The model under review builds one solid part; all positions refer to its coordinate system, in mm. Face numbers are marked on the shaded views. A direction names the side the tool comes from. Round coordinates to 2 decimals unless told otherwise and drop trailing zeros. Write each loop counter-clockwise with the first axis right and the second up, starting at its lowest first coordinate (ties: lowest second). Pieces come first, ordered by that corner, then holes. Notation, with made-up numbers: (46.25, 67) -> (80.25, 67) arc R23 ccw to (80.25, 81) -> close; hole circle Ø2 at (-21.75, 5). An arc over 180 degrees is marked (long way). Return JSON: item names as keys, results as strings. Group by question number.
1. Tool access review of the marked faces 1 and 2: name each direction out of +Z, -Z, +X, -X, +Y, -Y from which nothing blocks a thin tool from reaching the whole face with its end or side.
2. Take a section at A-A, the plane x = -16. Write out the cut boundary in (y, z).
3. Take a section at C-C, the plane x = -9. Write out the cut boundary in (y, z).
4. Take a section at B-B, the plane y = 15.5. Write out the cut boundary in (x, z).
5. Take a section at D-D, the plane z = 55.5. Write out the cut boundary in (x, y).
6. Clearance check with flat-ended pins moving along their axes: P1, Ø1.5, axis at y = 2, z = 15.5, coming from the +X side; P2, Ø10, axis at x = 13.5, z = 36.5, coming from the -Y side; P3, Ø5, axis at y = 10, z = 28.5, coming from the -X side. State where each tip first meets the part, or that it passes through.
7. For line 1 along Y through (x, z) = (-18.5, 3); line 2 along Z through (x, y) = (-18, -6.5); line 3 along X through (y, z) = (12.5, 23.5), list the stretches that pass through material, from the lowest coordinate up. Write a range as from..to.
8. Mouldability with a two-part tool opening along X and no side actions: class the marked faces 3, 4, 5 and 6 as pulls with the +X half, pulls with the -X half, needs draft (parallel to the pull), parting line crosses it, or undercut.
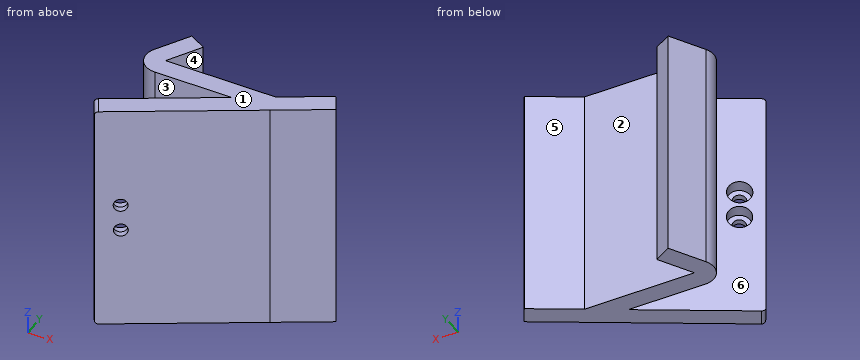
from build123d import *

# Parameters (mm, degrees)
SKETCH_1_W                          = 30
SKETCH_1_H                          = 5
EXTRUDE_1_DEPTH                     = 60
EXTRUDE_2_DEPTH                     = 60
EXTRUDE_3_DEPTH                     = 60
EXTRUDE_4_DEPTH                     = 60
HOLE_WIZARD_1_D                     = 3.4
HOLE_WIZARD_1_CBORE_D               = 6
HOLE_WIZARD_1_CBORE_DEPTH           = 3.4
HOLE_WIZARD_1_ON_FACE_2_D           = 3.4
HOLE_WIZARD_1_ON_FACE_2_CBORE_D     = 6
HOLE_WIZARD_1_ON_FACE_2_CBORE_DEPTH = 3.4
CUT_EXTRUDE_1_DEPTH                 = 60
CUT_EXTRUDE_2_DEPTH                 = 60


with BuildPart() as part:
    # Sketch 1 → Extrude 1 (new body)
    with BuildSketch(Plane.XY):
        with Locations((-4.245283019, 8.79713097)):
            Rectangle(SKETCH_1_W, SKETCH_1_H)
    extrude(amount=EXTRUDE_1_DEPTH)



with BuildPart() as body_2:
    # Sketch 2 → Extrude 2 (new body)
    with BuildSketch(Plane.XY.offset(60)):
        Polygon((-19.245283019, 11.29713097), (-14.245283019, 19.957385008), (-18.575410038, 22.457385008), (-23.575410038, 13.79713097), align=None)
    extrude(amount=-EXTRUDE_2_DEPTH)


with BuildPart() as part_1:
    add(part.part)

    add(body_2.part)  # Extrude 3 merges body 2
    # Sketch 3 → Extrude 3 (add)
    with BuildSketch(Plane.XY.offset(60)):
        with BuildLine():
            Line((-23.575410038, 13.79713097), (-19.245283019, 11.29713097))
            Line((-19.245283019, 11.29713097), (-19.245283019, 6.29713097))
            ThreePointArc((-19.245283019, 6.29713097), (-23.575410038, 8.79713097), (-23.575410038, 13.79713097))
        make_face()
    extrude(amount=-EXTRUDE_3_DEPTH)

    # Sketch 4 → Extrude 4 (add)
    with BuildSketch(Plane.XY.offset(60)):
        Polygon((10.754716981, 6.29713097), (-23.88629917, -13.70286903), (-26.38629917, -9.372742011), (8.254716981, 10.627257989), (21.245098038, 18.127257989), (23.745098038, 13.79713097), align=None)
    extrude(amount=-EXTRUDE_4_DEPTH)

    # Hole Wizard 1 (through all)
    with Locations(Plane(origin=(-21.157984096, -6.354172895, 26.500098518), x_dir=(0.866025403784, 0.5, 0), z_dir=(-0.5, 0.866025403784, 0))):
        with Locations((0, 0)):
            CounterBoreHole(HOLE_WIZARD_1_D / 2, HOLE_WIZARD_1_CBORE_D / 2, HOLE_WIZARD_1_CBORE_DEPTH)

    # Hole Wizard 1 on face 2 (through all)
    with Locations(Plane(origin=(-21.190146748, -6.372742011, 33.5), x_dir=(0.866025302838, 0.500000174844, 0), z_dir=(-0.500000174844, 0.866025302838, 0))):
        with Locations((0, 0)):
            CounterBoreHole(HOLE_WIZARD_1_ON_FACE_2_D / 2, HOLE_WIZARD_1_ON_FACE_2_CBORE_D / 2, HOLE_WIZARD_1_ON_FACE_2_CBORE_DEPTH)

    # Sketch 7 → Cut-Extrude 1 (cut)
    with BuildSketch(Plane(origin=(-2.53805845, 4.396046189, 0), x_dir=(0.8660254037844416, 0.499999999999995, 0), z_dir=(-0.499999999999995, 0.8660254037844416, 0))):
        with BuildLine():
            Line((-26.537576399, 0), (-27.537576399, 0))
            Line((-27.537576399, 0), (-27.537576399, -1))
            ThreePointArc((-27.537576399, -1), (-27.24468318, -0.292893219), (-26.537576399, 0))
        make_face()
    extrude(amount=-CUT_EXTRUDE_1_DEPTH, mode=Mode.SUBTRACT)

    # Sketch 9 → Cut-Extrude 2 (cut)
    with BuildSketch(Plane(origin=(-2.53805845, 4.396046189, 0), x_dir=(0.8660254037844416, 0.499999999999995, 0), z_dir=(-0.499999999999995, 0.8660254037844416, 0))):
        with BuildLine():
            Line((-27.537576399, -59), (-27.537576399, -60))
            Line((-27.537576399, -60), (-26.537576399, -60))
            ThreePointArc((-26.537576399, -60), (-27.24468318, -59.707106781), (-27.537576399, -59))
        make_face()
    extrude(amount=-CUT_EXTRUDE_2_DEPTH, mode=Mode.SUBTRACT)


solid = part_1.part
Output:
{
 "1": {"face 1": "+Z, +X, -X, +Y, -Y", "face 2": "+Z, -Z"},
 "2": {"outline": "(-9.15, 0) -> (-3.38, 0) -> (-3.38, 60) -> (-9.15, 60) -> close; (6.3, 0) -> (11.3, 0) -> (11.3, 60) -> (6.3, 60) -> close; (16.92, 0) -> (20.97, 0) -> (20.97, 60) -> (16.92, 60) -> close"},
 "3": {"outline": "(-5.11, 0) -> (0.67, 0) -> (0.67, 60) -> (-5.11, 60) -> close; (6.3, 0) -> (11.3, 0) -> (11.3, 60) -> (6.3, 60) -> close"},
 "4": {"outline": "(-22.59, 0) -> (-16.82, 0) -> (-16.82, 60) -> (-22.59, 60) -> close; (16.69, 0) -> (22.76, 0) -> (22.76, 60) -> (16.69, 60) -> close"},
 "5": {"outline": "(-26.39, -9.37) -> (-23.89, -13.7) -> (23.75, 13.8) -> (21.25, 18.13) -> (9.41, 11.3) -> (-19.25, 11.3) -> (-14.25, 19.96) -> (-18.58, 22.46) -> (-23.58, 13.8) arc R5 ccw to (-19.25, 6.3) -> (0.75, 6.3) -> close"},
 "6": {"P1": "stops at x = 4.61", "P2": "stops at y = 5", "P3": "stops at x = -24.25"},
 "7": {"line 1": "y = -10.59..-4.82, 6.3..11.3, 12.59..22.41", "line 2": "z = 0..25.12, 27.88..32.19, 34.81..60", "line 3": "x = -24.1..-18.55, 11.5..21.5"},
 "8": {"face 3": "needs draft", "face 4": "undercut", "face 5": "undercut", "face 6": "pulls with the -X half"}
}
